Design review of the part built by this model. Coordinates are the model's own, in mm. A direction names the side the tool comes from. Give positions to 0.01 mm unless a question says otherwise; leave off trailing zeros. Loops run counter-clockwise (first coordinate to the right, second up) from the corner with the lowest first, then second, coordinate; pieces in that order, holes last. Notation, with made-up numbers: (3, -23.75) -> (20, -23.75) arc R32 ccw to (20, 11.25) -> close; hole circle Ø4 at (18, 57.25). An arc over 180 degrees is marked (long way). Use a Markdown table: item, result. Add a question column.
1. For faces 4 (the cylindrical face through (25.65, -8.1, -2.55)), 5 (the cylindrical face through (14.23, -8.1, -2.55)), 6 (the cylindrical face through (-19.6, -3.65, -8.8)), 7 (the cylindrical face through (-3.65, 19.6, -8.8)), list the 3-axis set-ups (+Z, -Z, +X, -X, +Y, -Y) from which the entire face can be reached by the end or side of a thin tool; tool diameter is ignored.
2. Add section D-D (z = 1). Count the separate pieces of the cut face and the enclosed holes in it, and give its area (3 significant figures).
3. Add section A-A (x = 0). State the section outline as (y, z) points (3 decimals), and give its area (3 significant figures).
4. Draft analysis for pull direction X (two halves, no side actions). For faces 1 (the flat face through (-30.95, 5, 2)), 2 (the cylindrical face through (-14.23, 8.1, -2.55)), 3 (the cylindrical face through (-25.65, 8.1, -2.55)), state which applies: pulls with the +X half, pulls with the -X half, needs draft (parallel to the pull), parting line crosses it, or undercut.
5. For pin 1 Ø5 at (x, z) = (-3, -4.5) entering from -Y; pin 2 Ø1 at (x, y) = (-18, 8) entering from +Z; pin 3 Ø8 at (x, z) = (0, 0) entering from +Y, all flat-tipped, find the tip position at first contact; note any pin that passes through.
6. Add section C-C (x = 11). State the section outline as (y, z) points (3 decimals), and give its area (3 significant figures).
7. Add section B-B (y = 25.5). State the section outline as (x, z) points, and give its area (3 significant figures).
8. To check wall thickness, follow line 1 (Z direction, x = 0, y = 5) (3 decimals); line 2 (Z direction, x = 0, y = 14); line 3 (Y direction, x = 9, z = 0) (3 decimals). State the ranges of each line that lie inside material, in increasing order.
```python
from build123d import *

# Parameters (mm, degrees)
SKETCH2_R           = 9.525
EXTRUDE1_DEPTH      = 17.526
SKETCH15_R          = 9.525
BOSS_EXTRUDE1_DEPTH = 13.4239
SKETCH16_R          = 4.9657
CUT_EXTRUDE1_DEPTH  = 34.754222847
CIRPATTERN1_COUNT   = 3
CIRPATTERN1_ANGLE   = 180
SKETCH17_R          = 4.9657
CUT_EXTRUDE2_DEPTH  = 70.858479622
CUT_EXTRUDE3_REACH  = 53.835
SKETCH18_R          = 4.9657


with BuildPart() as part:
    # Sketch2 → Extrude1 (new body)
    with BuildSketch(Plane(origin=(-30.9499, 0, 0), x_dir=(0, 0, -1), z_dir=(1, 0, 0))):
        Circle(SKETCH2_R)
    extrude(amount=EXTRUDE1_DEPTH)

    # Sketch5 → Cut-Revolve1 (revolve, cut)
    with BuildSketch(Plane.XY):
        Polygon((-27.256291687, 8.493888504), (-24.081291687, 8.493888504), (-23.050180191, 9.525), (-30.9499, 9.525), (-30.9499, 5.710555), align=None)
        Polygon((-13.4239, 8.493888504), (-15.0114, 8.493888504), (-16.042511496, 9.525), (-13.4239, 9.525), align=None)
    revolve(axis=Axis((0, 0, 0), (-1, 0, 0)), mode=Mode.SUBTRACT)

    # Sketch15 → Boss-Extrude1 (add)
    with BuildSketch(Plane(origin=(-13.4239, 0, 0), x_dir=(0, 0, -1), z_dir=(1, 0, 0))):
        with Locations(Location((0, 0, 0), (0, 0, 90))):
            Circle(SKETCH15_R)
    extrude(amount=BOSS_EXTRUDE1_DEPTH)

    # Sketch16 → Cut-Extrude1 (cut, through all)
    with BuildSketch(Plane(origin=(0, 0, 0), x_dir=(0, 0, -1), z_dir=(1, 0, 0))):
        Circle(SKETCH16_R)
    extrude(amount=-CUT_EXTRUDE1_DEPTH, mode=Mode.SUBTRACT)


with BuildPart() as cirpattern1_1:
    # CirPattern1: pattern copy
    add(part.part.rotate(Axis((0, 0, 0), (0, 0, -1)), 1 * CIRPATTERN1_ANGLE / (CIRPATTERN1_COUNT - 1)))

    # Sketch17 → Cut-Extrude2 (cut, through all)
    with BuildSketch(Plane.ZY.offset(30.9499)):
        with Locations(Location((0, 0, 0), (0, 0, 180))):
            Circle(SKETCH17_R)
    extrude(amount=-CUT_EXTRUDE2_DEPTH, mode=Mode.SUBTRACT)


with BuildPart() as cirpattern1_2:
    # CirPattern1: pattern copy
    add(part.part.rotate(Axis((0, 0, 0), (0, 0, -1)), 2 * CIRPATTERN1_ANGLE / (CIRPATTERN1_COUNT - 1)))


with BuildPart() as cirpattern1_1_1:
    add(cirpattern1_1.part)

    # Combine1: union part, CirPattern1_2
    add(part.part)
    add(cirpattern1_2.part)

    # Sketch18 → Cut-Extrude3 (cut, up to next)
    with BuildSketch(Plane(origin=(0, 30.9499, 0), x_dir=(1, 0, 0), z_dir=(0, 1, 0)), mode=Mode.PRIVATE) as cut_extrude3_sk1:
        with Locations(Location((0, 0, 0), (0, 0, 90))):
            Circle(SKETCH18_R)
    cut_extrude3_tool1 = extrude(cut_extrude3_sk1.sketch, amount=-CUT_EXTRUDE3_REACH, mode=Mode.PRIVATE) & cirpattern1_1_1.part
    add(cut_extrude3_tool1.solids().sort_by_distance((0, 30.9499, 0))[0], mode=Mode.SUBTRACT)


solid = cirpattern1_1_1.part
```
Taken from the geometry:
| question | item | result |
|---|---|---|
| 1 | face 4 | +X |
| 1 | face 5 | none |
| 1 | face 6 | -X |
| 1 | face 7 | +Y |
| 2 | separate pieces | 3 |
| 2 | enclosed holes | 0 |
| 2 | area | 633 mm^2 |
| 3 | outline | (0, -9.525) -> (13.424, -9.525) -> (13.424, -8.494) -> (15.011, -8.494) -> (16.043, -9.525) -> (23.05, -9.525) -> (24.081, -8.494) -> (27.256, -8.494) -> (30.95, -5.711) -> (30.95, -4.966) -> (0, -4.966) arc R4.966 cw to (0, 4.966) -> (30.95, 4.966) -> (30.95, 5.711) -> (27.256, 8.494) -> (24.081, 8.494) -> (23.05, 9.525) -> (16.043, 9.525) -> (15.011, 8.494) -> (13.424, 8.494) -> (13.424, 9.525) -> (0, 9.525) arc R9.525 ccw to start |
| 3 | area | 356 mm^2 |
| 4 | face 1 | pulls with the -X half |
| 4 | face 2 | undercut |
| 4 | face 3 | needs draft |
| 5 | pin 1 | stops at y = -9.31 |
| 5 | pin 2 | stops at z = 5.87 |
| 5 | pin 3 | stops at y = -2.94 |
| 6 | outline | circle Ø19.05 at (0, 0); hole circle Ø9.931 at (0, 0) |
| 6 | area | 208 mm^2 |
| 7 | outline | circle Ø16.99 at (0, 0); hole circle Ø9.93 at (0, 0) |
| 7 | area | 149 mm^2 |
| 8 | line 1 | z = -9.525 to -4.966, 4.966 to 9.525 |
| 8 | line 2 | z = -8.49 to -4.97, 4.97 to 8.49 |
| 8 | line 3 | y = -9.525 to -4.966, 4.966 to 13.424, 15.518 to 23.575 |
